Verification items for this drawing (mm, ordinates from the low corner). Round coordinates to 2 decimals unless told otherwise and drop trailing zeros. Loops run counter-clockwise (first coordinate to the right, second up) from the corner with the lowest first, then second, coordinate; pieces in that order, holes last. Notation, with made-up numbers: M -13.5,27.25 L 29.5,27.25 A25 cw 29.5,43.25 Z; hole C 30.5,-21 d7. An arc over 180 degrees is marked long. Answer as CSV lines item,"result".
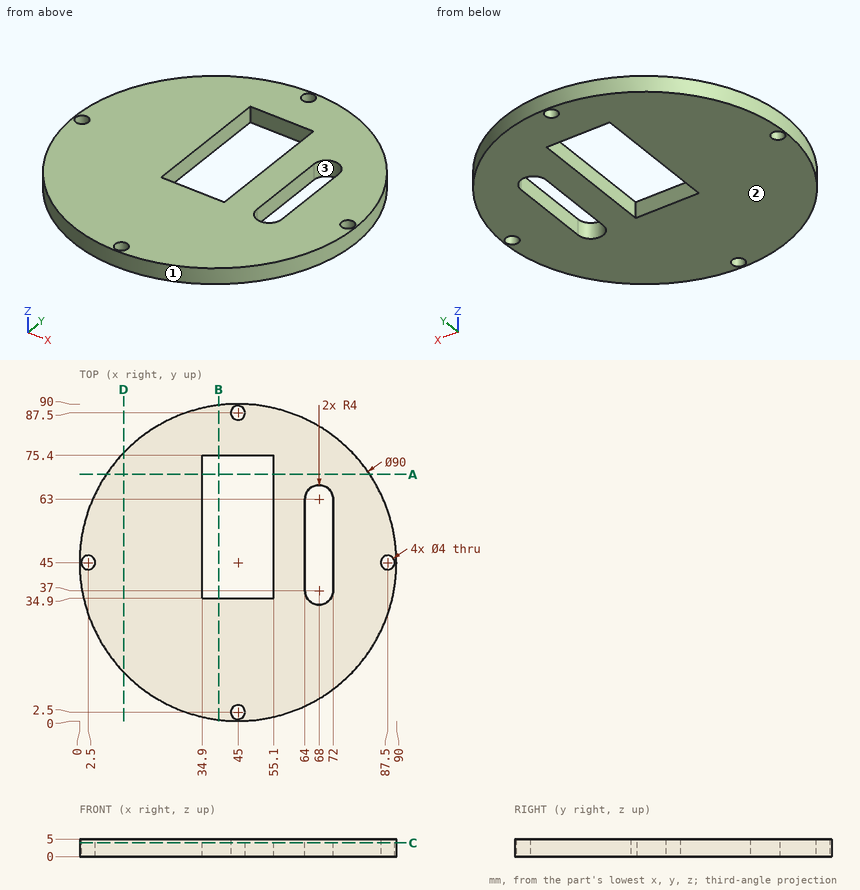
1) Draft check along X on the marked faces 1, 2 and 3. Enter one of: +X half, -X half, draft (parallel to the pull), parting line (faces both ways), or undercut.
Here are the results:
face 1,"parting line"
face 2,"draft"
face 3,"undercut"
2) Go/stop test with flat-tipped pins: pin 1 (3 mm diameter, centred on y = 65, z = 2, fed in from +X); pin 2 (4 mm diameter, centred on x = 24, y = 32, fed in from -Z); pin 3 (2.5 mm diameter, centred on y = 51, z = 2, fed in from -X); pin 4 (1.5 mm diameter, centred on y = 16.5, z = 3, fed in from +X). Record where each tip stops, or that it passes through.
Here are the results:
pin 1,"stops at x = 86.02"
pin 2,"stops at z = 0"
pin 3,"stops at x = 0.25"
pin 4,"stops at x = 80.43"
3) Material ranges on probe 1 along Y at (x, z) = (45, 3.7); probe 2 along X at (y, z) = (57, 4.15); probe 3 along X at (y, z) = (36.5, 1.15), recorded low to high.
Here are the results:
probe 1,"y = 0 to 0.5, 4.5 to 34.9, 75.4 to 85.5, 89.5 to 90"
probe 2,"x = 1.63 to 34.9, 55.1 to 64, 72 to 88.37"
probe 3,"x = 0.81 to 34.9, 55.1 to 64.03, 71.97 to 89.19"
4) Section check C-C (z = 3.9). Record the cut outline in (x, y).
Here are the results:
outline,"C 45,45 d90; hole C 2.5,45 d4; hole M 34.9,34.9 L 55.1,34.9 L 55.1,75.4 L 34.9,75.4 Z; hole C 45,2.5 d4; hole C 45,87.5 d4; hole M 64,37 A4 ccw 72,37 L 72,63 A4 ccw 64,63 Z; hole C 87.5,45 d4"
5) Section check A-A (y = 70). Record the cut outline in (x, z).
Here are the results:
outline,"M 7.58,0 L 34.9,0 L 34.9,5 L 7.58,5 Z; M 55.1,0 L 82.42,0 L 82.42,5 L 55.1,5 Z"
6) Section check B-B (x = 39.5). Record the cut outline in (y, z), plus the area to 3 significant figures.
Here are the results:
outline,"M 0.34,0 L 34.9,0 L 34.9,5 L 0.34,5 Z; M 75.4,0 L 89.66,0 L 89.66,5 L 75.4,5 Z"
area,"244 mm^2"
7) Section check D-D (x = 12.5). Record the cut outline in (y, z), plus the area to 3 significant figures.
Here are the results:
outline,"M 13.88,0 L 76.12,0 L 76.12,5 L 13.88,5 Z"
area,"311 mm^2"
